Geometry check sheet. Reference: the model listing, model coordinates, mm. Coordinates: 2 decimals unless noted, no trailing zeros. Loops run counter-clockwise (first coordinate to the right, second up) from the corner with the lowest first, then second, coordinate; pieces in that order, holes last. Notation, with made-up numbers: M -7.5,-7 L 20.5,-7 A20 cw 20.5,21 Z; hole C -24,64 d8. An arc over 180 degrees is marked long. Use CSV: the item, a comma, the result in double quotes.
```python
from build123d import *

# Parameters (mm, degrees)
BOSS_EXTRUDE1_DEPTH = 95.25
SKETCH3_R           = 38.1
CUT_EXTRUDE1_DEPTH  = 43.539324096
SKETCH4_R           = 3.175
CUT_EXTRUDE2_DEPTH  = 43.539324096


with BuildPart() as part:
    # Sketch2 → Boss-Extrude1 (new body)
    with BuildSketch(Plane.XY):
        Polygon((6.664773782, 3.320633799), (0.338937449, 3.874072765), (36.666498884, 419.1), (42.992335217, 418.546561034), align=None)
    extrude(amount=BOSS_EXTRUDE1_DEPTH)

    # Sketch3 → Cut-Extrude1 (cut, through all)
    with BuildSketch(Plane(origin=(0, 0, 0), x_dir=(0, 0, 1), z_dir=(-0.996194698, 0.087155743, 0))):
        with Locations((47.625, 373.075893914)):
            Circle(SKETCH3_R)
    extrude(amount=-CUT_EXTRUDE1_DEPTH, mode=Mode.SUBTRACT)

    # Sketch4 → Cut-Extrude2 (cut, through all)
    with BuildSketch(Plane(origin=(0, 0, 0), x_dir=(0, 0, 1), z_dir=(-0.996194698, 0.087155743, 0))):
        with Locations((9.525, 19.763871094)):
            Circle(SKETCH4_R)
        with Locations((85.725, 19.763871094)):
            Circle(SKETCH4_R)
    extrude(amount=-CUT_EXTRUDE2_DEPTH, mode=Mode.SUBTRACT)


solid = part.part
```
1. Gauge pin test, flat end, axial feed: P1, Ø12, axis at x = 9.5, z = 50.5, coming from the -Y side. Record the tip position at first contact, or that the pin passes through.
The answers:
P1,"y = 3.32"
2. Section check D-D, the plane x = 18.5. Record the cut outline in (y, z).
The answers:
outline,"M 138.6,0 L 211.46,0 L 211.46,95.25 L 138.6,95.25 Z"
3. Section check C-C, the plane y = 321. Record the cut outline in (x, z).
The answers:
outline,"M 28.08,0 L 34.46,0 L 34.46,95.25 L 28.08,95.25 Z"
4. Section check B-B, the plane z = 46. Record the cut outline in (x, y).
The answers:
outline,"M 0.34,3.87 L 6.66,3.32 L 35.52,333.18 L 29.2,333.74 Z; M 35.83,409.58 L 42.16,409.02 L 42.99,418.55 L 36.67,419.1 Z"
5. Section check A-A, the plane z = 77.5. Record the cut outline in (x, y).
The answers:
outline,"M 0.34,3.87 L 6.66,3.32 L 36.78,347.55 L 30.45,348.1 Z; M 34.58,395.21 L 40.9,394.66 L 42.99,418.55 L 36.67,419.1 Z"
6. Release check for a two-part mould opening along Y. For faces 1 (the flat face through (14.21, 162.44, 46.96)), 2 (the cylindrical face through (4.735, 18.204, 12.458)), 3 (the flat face through (22, 212, 95.25)) record: +Y half, -Y half, draft (parallel to the pull), parting line (faces both ways), or undercut.
The answers:
face 1,"+Y half"
face 2,"undercut"
face 3,"draft"
7. Thickness scan on line 1 (X direction, y = 269, z = 64); line 2 (X direction, y = 123.5, z = 62); line 3 (Y direction, x = 39, z = 79.5). Record the ranges inside material, lowest first. Write a range as [from, to].
The answers:
line 1,"[23.53, 29.91]"
line 2,"[10.8, 17.18]"
line 3,"[392.04, 418.9]"
